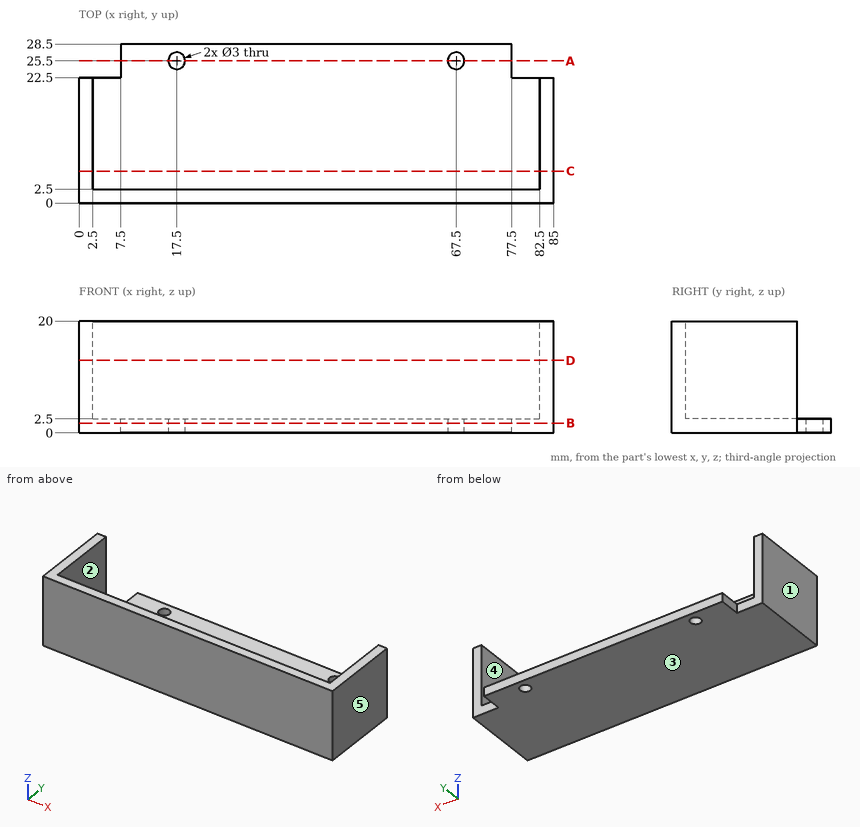
Geometry: see drawing. Coordinates: mm, zero at the bounding-box minimum. A direction names the side the tool comes from. Round coordinates to 2 decimals unless told otherwise and drop trailing zeros. Loops run counter-clockwise (first coordinate to the right, second up) from the corner with the lowest first, then second, coordinate; pieces in that order, holes last. Notation, with made-up numbers: (69.5, 28) -> (102.5, 28) arc R23 ccw to (102.5, 39) -> close; hole circle Ø11 at (-37.75, -0.5). An arc over 180 degrees is marked (long way). Write each question's results on one line, items separated by ' | '.
Item 1: Cut plane A-A on y = 25.5. Return the cut outline in (x, z).
Answers below:
outline: (7.5, 0) -> (16, 0) -> (16, 2.5) -> (7.5, 2.5) -> close; (19, 0) -> (66, 0) -> (66, 2.5) -> (19, 2.5) -> close; (69, 0) -> (77.5, 0) -> (77.5, 2.5) -> (69, 2.5) -> close
Item 2: Line query: probe 1 along X at (y, z) = (22, 16.25); probe 2 along Y at (x, z) = (67.5, 1.9); probe 3 along X at (y, z) = (25.75, 1.5). Output: solid intervals per line, ascending. Write a range as [from, to].
Answers below:
probe 1: x = [0, 2.5], [82.5, 85] | probe 2: y = [0, 24], [27, 28.5] | probe 3: x = [7.5, 16.02], [18.98, 66.02], [68.98, 77.5]
Item 3: Cut plane D-D on z = 13. Return the cut outline in (x, y).
Answers below:
outline: (0, 0) -> (85, 0) -> (85, 22.5) -> (82.5, 22.5) -> (82.5, 2.5) -> (2.5, 2.5) -> (2.5, 22.5) -> (0, 22.5) -> close
Item 4: Set-up query: the marked faces 4 and 5. Return all of +Z, -Z, +X, -X, +Y, -Y with unobstructed straight access to the full face (end or side cutting, diameter ignored); none if empty.
Answers below:
face 4: +Z, +Y | face 5: +Z, -Z, +X, +Y, -Y
Item 5: Pin query (flat end, axial travel): pin 1 Ø1.5 at (x, y) = (49, 7.5) entering from +Z; pin 2 Ø8 at (y, z) = (4.5, 16.5) entering from -X; pin 3 Ø2.5 at (x, y) = (17.5, 25.5) entering from -Z; pin 4 Ø9 at (x, z) = (40.5, 8) entering from +Y. Return the tip coordinate at first contact, or that it passes through.
Answers below:
pin 1: stops at z = 2.5 | pin 2: stops at x = 0 | pin 3: passes through | pin 4: stops at y = 2.5
Item 6: Cut plane C-C on y = 5.75. Return the cut outline in (x, z).
Answers below:
outline: (0, 0) -> (85, 0) -> (85, 20) -> (82.5, 20) -> (82.5, 2.5) -> (2.5, 2.5) -> (2.5, 20) -> (0, 20) -> close
Item 7: Cut plane B-B on z = 1.75. Return the cut outline in (x, y), and give its area (3 significant figures).
Answers below:
outline: (0, 0) -> (85, 0) -> (85, 22.5) -> (77.5, 22.5) -> (77.5, 28.5) -> (7.5, 28.5) -> (7.5, 22.5) -> (0, 22.5) -> close; hole circle Ø3 at (17.5, 25.5); hole circle Ø3 at (67.5, 25.5) | area: 2,320 mm²
Item 8: Pull-direction query (X, two-part tool) for the marked faces 1, 2 and 3; classes: pulls with the +X half, pulls with the -X half, needs draft (parallel to the pull), parting line crosses it, or undercut.
Answers below:
face 1: pulls with the -X half | face 2: undercut | face 3: needs draft
